```python
from build123d import *

# Parameters (mm, degrees)
SKETCH116_R     = 2.286
PAD042_DEPTH    = 6.35
SKETCH117_R     = 3.683
POCKET041_DEPTH = 2.54


with BuildPart() as part:
    # Sketch116 → Pad042 (new body)
    with BuildSketch(Plane.YZ):
        with BuildLine():
            Line((-86.423367, 0), (-104.021003, 30.48))
            Line((-104.021003, 30.48), (-62.282204, 17.844963))
            Line((-62.282204, 17.844963), (-57.965562, 0))
            Line((-64.816504, 0), (-57.965562, 0))
            ThreePointArc((-64.816504, 0), (-73.056938, 8.240434), (-81.297372, 0))
            Line((-86.423367, 0), (-81.297372, 0))
        make_face()
        with Locations((-79.389436, 12.7)):
            Circle(SKETCH116_R, mode=Mode.SUBTRACT)
        with Locations((-66.689436, 12.7)):
            Circle(SKETCH116_R, mode=Mode.SUBTRACT)
    pad042 = extrude(amount=PAD042_DEPTH)

    # Sketch117 → Pocket041 (cut)
    with BuildSketch(Plane.YZ.offset(6.35)):
        with Locations((-79.389436, 12.7)):
            Circle(SKETCH117_R)
        with Locations((-66.689436, 12.7)):
            Circle(SKETCH117_R)
    pocket041 = extrude(amount=-POCKET041_DEPTH, mode=Mode.SUBTRACT)

    # Mirrored003: Pad042, Pocket041 across XY
    add(pad042.mirror(Plane.XY))
    add(pocket041.mirror(Plane.XY), mode=Mode.SUBTRACT)


with BuildPart() as part_1:
    # Body033 placement: moved
    add(part.part.moved(Location((11.049, 0, 0))))


solid = part_1.part
```
The model under review builds one solid part; all positions refer to its coordinate system, in mm. A direction names the side the tool comes from. Give positions to 0.01 mm unless a question says otherwise; leave off trailing zeros. Write each loop counter-clockwise with the first axis right and the second up, starting at its lowest first coordinate (ties: lowest second). Pieces come first, ordered by that corner, then holes. Notation, with made-up numbers: M -37.5,89.25 L -8.5,89.25 A15 cw -8.5,103.25 Z; hole C 1,47.25 d3. An arc over 180 degrees is marked long. Answer in a Markdown table with one row per item.
Item 1: Draft analysis for pull direction Z (two halves, no side actions). For faces 1 (the face through (14.859, -79, -10)), 2 (the face through (14.18, -60.154, -9.047)), 3 (the face through (14.18, -83.44, 24.25)), state which applies: +Z half, -Z half, draft (parallel to the pull), parting line (faces both ways), or undercut.
Check sheet entries:
| item | result |
|---|---|
| face 1 | undercut |
| face 2 | -Z half |
| face 3 | +Z half |
Item 2: For line 1 along Z through (x, y) = (15, -78); line 2 along Y through (x, z) = (16.15, -12.7); line 3 along Z through (x, y) = (14.5, -68), list the stretches that pass through material, from the lowest coordinate up.
Check sheet entries:
| item | result |
|---|---|
| line 1 | -22.6 to -16.11, -9.29 to -6.59, 6.59 to 9.29, 16.11 to 22.6 |
| line 2 | -93.76 to -83.07, -75.71 to -70.37, -63.01 to -61.04 |
| line 3 | -19.58 to -14.57, -10.83 to -6.51, 6.51 to 10.83, 14.57 to 19.58 |
Item 3: Add section A-A on x = 15.5. Give the boundary of the cut face in (y, z).
Check sheet entries:
| item | result |
|---|---|
| outline | M -104.02,-30.48 L -62.28,-17.84 L -57.97,0 L -62.28,17.84 L -104.02,30.48 L -86.42,0 Z; hole C -79.39,-12.7 d7.37; hole C -79.39,12.7 d7.37; hole C -73.06,0 d16.48; hole C -66.69,-12.7 d7.37; hole C -66.69,12.7 d7.37 |
Item 4: Add section C-C on z = 12.7. Give the boundary of the cut face in (x, y), plus the area to 3 significant figures.
Check sheet entries:
| item | result |
|---|---|
| outline | M 11.05,-93.76 L 17.4,-93.76 L 17.4,-83.07 L 14.86,-83.07 L 14.86,-81.68 L 11.05,-81.68 Z; M 11.05,-77.1 L 14.86,-77.1 L 14.86,-75.71 L 17.4,-75.71 L 17.4,-70.37 L 14.86,-70.37 L 14.86,-68.98 L 11.05,-68.98 Z; M 11.05,-64.4 L 14.86,-64.4 L 14.86,-63.01 L 17.4,-63.01 L 17.4,-61.04 L 11.05,-61.04 Z |
| area | 136 mm2 |
Item 5: Add section B-B on y = -94.5. Give the boundary of the cut face in (x, z).
Check sheet entries:
| item | result |
|---|---|
| outline | M 11.05,-27.6 L 17.4,-27.6 L 17.4,-13.99 L 11.05,-13.99 Z; M 11.05,13.99 L 17.4,13.99 L 17.4,27.6 L 11.05,27.6 Z |
Item 6: Add section D-D on z = 6. Give the boundary of the cut face in (x, y).
Check sheet entries:
| item | result |
|---|---|
| outline | M 11.05,-89.89 L 17.4,-89.89 L 17.4,-78.71 L 11.05,-78.71 Z; M 11.05,-67.41 L 17.4,-67.41 L 17.4,-59.42 L 11.05,-59.42 Z |
Item 7: Tool access review of faces 4 (the face through (16.147, -75.987, 11.289)), 5 (the face through (14.18, -60.154, 9.047)), 6 (the face through (14.18, -95.1, -15.03)): name each direction out of +Z, -Z, +X, -X, +Y, -Y from which nothing blocks a thin tool from reaching the whole face with its end or side.
Check sheet entries:
| item | result |
|---|---|
| face 4 | +X |
| face 5 | +Z, +X, -X, +Y |
| face 6 | +X, -X, -Y |
Item 8: For P1, Ø6, axis at y = -79.39, z = -12.7, coming from the +X side; P2, Ø8, axis at y = -67, z = 11.5, coming from the +X side; P3, Ø4.5, axis at y = -66.69, z = -12.7, coming from the +X side; P4, Ø2, axis at x = 13.5, z = -9, coming from the +Y side, all flat-tipped, find the tip position at first contact; note any pin that passes through.
Check sheet entries:
| item | result |
|---|---|
| P1 | x = 14.86 |
| P2 | x = 17.4 |
| P3 | through |
| P4 | y = -59.9 |
